CAD build for the part. Positions are in the model's coordinates, mm. A direction names the side the tool comes from. Give positions to 0.01 mm unless a question says otherwise; leave off trailing zeros. Write each loop counter-clockwise with the first axis right and the second up, starting at its lowest first coordinate (ties: lowest second). Pieces come first, ordered by that corner, then holes. Notation, with made-up numbers: (34.5, 42.5) - (46.5, 42.5) arc R21 cw to (46.5, 48.5) - close; hole circle Ø11 at (-17, -33). An arc over 180 degrees is marked (long way). Put each result on its own line as item: value. Start each with the question number.
1. Cut at A-A on y = -69. List the corners of the cut face in (x, z).
2. Cut at D-D on x = -2. List the corners of the cut face in (y, z), and give its area (3 significant figures).
3. Tool access for faces 4 (the cylindrical face through (45.2, -64.8, 7.6)), 5 (the flat face through (-5.3, -79.412, 83.3)), 6 (the flat face through (13.487, -27, 28)), 7 (the flat face through (-7, -39, 6.962)), 8 (the flat face through (-10, -41.808, 31)): list every direction of +Z, -Z, +X, -X, +Y, -Y with a clear straight run to the whole face (end or side of a thin tool).
4. Wall check: line 1 (X direction, y = -46, z = 75); line 2 (Z direction, x = 6, y = -47); line 3 (Z direction, x = 39, y = -31.5). Give the ranges that are in metal, low to high.
5. Drop flat-ended pins along their axis: pin 1 (3 mm diameter, centred on x = 18.5, z = 26.5, fed in from -Y); pin 2 (6 mm diameter, centred on x = -50, y = -60.5, fed in from +Z); pin 3 (10 mm diameter, centred on x = 31.5, y = -38.5, fed in from +Z); pin 4 (12 mm diameter, centred on x = -32.5, z = 56.5, fed in from -Y). Give the stop position or say it passes through.
6. Cut at B-B on y = -61. List the corners of the cut face in (x, z), and give its area (3 significant figures).
7. Cut at C-C on z = 80. List the corners of the cut face in (x, y).
8. Mould opens along Z. For faces 1 (the flat face through (-9, -31.808, 31)), 2 (the flat face through (-7, 0, 9)), 3 (the flat face through (38, -39, 0)) say: +Z half, -Z half, draft (parallel to the pull), parting line (faces both ways), or undercut.
from build123d import *

# Parameters (mm, degrees)
F1_DEPTH  = 80
F2_R      = 5
F3_DEPTH  = 25
F5_DEPTH  = 60
F6_R      = 35
F7_DEPTH  = 33
F8_DEPTH  = 25
F9_R      = 25
F10_DEPTH = 52.6
F11_R     = 25
F12_DEPTH = 52.6
F14_DEPTH = 25


with BuildPart() as f1:
    # F0 (on Front) → F1 (new body)
    with BuildSketch(Plane.XZ):
        Polygon((-66.513142, 0), (-36.513142, 0), (-36.513142, 6.962258), (23.486858, 6.962258), (23.486858, 0), (53.486858, 0), (53.486858, 15), (-66.513142, 15), align=None)
    extrude(amount=F1_DEPTH)

    # F2 (on face) → F3 (cut)
    with BuildSketch(Plane.XY.offset(15)):
        with Locations((42.486858, -11)):
            Circle(F2_R)
        with Locations((42.486858, -69)):
            Circle(F2_R)
        with Locations((-55.513142, -69)):
            Circle(F2_R)
        with Locations((-55.513142, -11)):
            Circle(F2_R)
    extrude(amount=-F3_DEPTH, mode=Mode.SUBTRACT)

    # F4 (on face) → F5 (join)
    with BuildSketch(Plane.XY.offset(15)):
        Polygon((23.486858, -54.41226), (23.486858, -21.807771), (13.486858, -21.807771), (13.486858, -31.807771), (-32.013142, -31.807771), (-32.013142, -41.807771), (13.486858, -41.807771), (13.486858, -54.41226), align=None)
    extrude(amount=F5_DEPTH)

    # F6 (on face) → F7 (join)
    with BuildSketch(Plane.XZ.offset(54.41226)):
        with Locations((18.486858, 75)):
            Circle(F6_R)
    extrude(amount=-F7_DEPTH)

    # F6 (on face) → F8 (join)
    with BuildSketch(Plane.XZ.offset(54.41226)):
        with Locations((18.486858, 75)):
            Circle(F6_R)
    extrude(amount=F8_DEPTH)

    # F9 (on face) → F10 (cut)
    with BuildSketch(Plane.XZ.offset(79.41226)):
        with Locations((18.486858, 75)):
            Circle(F9_R)
    extrude(amount=-F10_DEPTH, mode=Mode.SUBTRACT)

    # F11 (on face) → F12 (cut)
    with BuildSketch(Plane(origin=(0, -21.41226, 0), x_dir=(-1, 0, 0), z_dir=(0, 1, 0))):
        with Locations((-18.486858, 75)):
            Circle(F11_R)
    extrude(amount=-F12_DEPTH, mode=Mode.SUBTRACT)

    # F13 (on face) → F14 (cut)
    with BuildSketch(Plane.XZ.offset(41.807771)):
        Polygon((-32.013142, 15), (-16.513142, 75), (-32.013142, 75), align=None)
    extrude(amount=-F14_DEPTH, mode=Mode.SUBTRACT)


solid = f1.part
Report:
1. outline: (-66.51, 0) - (-60.51, 0) - (-60.51, 15) - (-66.51, 15) - close; (-50.51, 0) - (-36.51, 0) - (-36.51, 6.96) - (23.49, 6.96) - (23.49, 0) - (37.49, 0) - (37.49, 15) - (-50.51, 15) - close; circle Ø70 at (18.49, 75); (47.49, 0) - (53.49, 0) - (53.49, 15) - (47.49, 15) - close; hole circle Ø50 at (18.49, 75)
2. outline: (-80, 6.96) - (0, 6.96) - (0, 15) - (-31.81, 15) - (-31.81, 46.62) - (-21.41, 46.62) - (-21.41, 60.67) - (-79.41, 60.67) - (-79.41, 46.62) - (-41.81, 46.62) - (-41.81, 15) - (-80, 15) - close; (-79.41, 89.33) - (-21.41, 89.33) - (-21.41, 103.38) - (-79.41, 103.38) - close
2. area: 2,590 mm²
3. face 4: -Z
3. face 5: +Z, +X, -X, -Y
3. face 6: -X, +Y
3. face 7: -Z, +Y, -Y
3. face 8: -X, -Y
4. line 1: x = -16.51 to -6.51, 43.49 to 53.49
4. line 2: z = 6.96 to 15, 42.3 to 53.34, 96.66 to 107.7
4. line 3: z = 0 to 15, 46.64 to 60.71, 89.29 to 103.36
5. pin 1: stops at y = -54.41
5. pin 2: stops at z = 15
5. pin 3: stops at z = 109.07
5. pin 4: passes through
6. outline: (-66.51, 0) - (-36.51, 0) - (-36.51, 6.96) - (23.49, 6.96) - (23.49, 0) - (53.49, 0) - (53.49, 15) - (-66.51, 15) - close; circle Ø70 at (18.49, 75); hole circle Ø50 at (18.49, 75)
6. area: 3,270 mm²
7. outline: (-16.15, -79.41) - (-6.01, -79.41) - (-6.01, -21.41) - (-16.15, -21.41) - close; (42.98, -79.41) - (53.13, -79.41) - (53.13, -21.41) - (42.98, -21.41) - close
8. face 1: undercut
8. face 2: draft
8. face 3: -Z half
